For this review, take the finished solid that the model builds, in its own axes (mm). A direction names the side the tool comes from. Round coordinates to 2 decimals unless told otherwise and drop trailing zeros. Write each loop counter-clockwise with the first axis right and the second up, starting at its lowest first coordinate (ties: lowest second). Pieces come first, ordered by that corner, then holes. Notation, with made-up numbers: M 65.5,41.25 L 92.5,41.25 A22 ccw 92.5,70.25 Z; hole C 57,87 d10. An arc over 180 degrees is marked long. Answer in a Markdown table with one row per item.
```python
from build123d import *

# Parameters (mm, degrees)
SKETCH1_R           = 3.25
SKETCH1_R_2         = 2.25
BOSS_EXTRUDE1_DEPTH = 4.5
SKETCH2_R           = 8.5
SKETCH2_R_2         = 0.85
SKETCH2_R_3         = 1
BOSS_EXTRUDE2_DEPTH = 2


with BuildPart() as part:
    # Sketch1 → Boss-Extrude1 (new body)
    with BuildSketch(Plane.XY):
        Circle(SKETCH1_R)
        Circle(SKETCH1_R_2, mode=Mode.SUBTRACT)
    extrude(amount=BOSS_EXTRUDE1_DEPTH)

    # Sketch2 → Boss-Extrude2 (add)
    with BuildSketch(Plane(origin=(0, 0, 0), x_dir=(-1, 0, 0), z_dir=(0, 0, -1))):
        Circle(SKETCH2_R)
        Circle(SKETCH2_R_2, mode=Mode.SUBTRACT)
        with Locations((-6, 0)):
            Circle(SKETCH2_R_3, mode=Mode.SUBTRACT)
        with Locations((0, 6)):
            Circle(SKETCH2_R_3, mode=Mode.SUBTRACT)
        with Locations((6, 0)):
            Circle(SKETCH2_R_3, mode=Mode.SUBTRACT)
        with Locations((0, -6)):
            Circle(SKETCH2_R_3, mode=Mode.SUBTRACT)
    extrude(amount=-BOSS_EXTRUDE2_DEPTH)


solid = part.part
```
Q1. Take a section at A-A (y = -6). State the section outline as (x, z) points.
Found:
| item | result |
|---|---|
| outline | M -6.02,0 L -1,0 L -1,2 L -6.02,2 Z; M 1,0 L 6.02,0 L 6.02,2 L 1,2 Z |
Q2. Take a section at C-C (z = 0.75). State the section outline as (x, y) points, then the cut area to 3 significant figures.
Found:
| item | result |
|---|---|
| outline | C 0,0 d17; hole C -6,0 d2; hole C 0,-6 d2; hole C 0,6 d2; hole C 0,0 d1.7; hole C 6,0 d2 |
| area | 212 mm² |
Q3. Mouldability with a two-part tool opening along X and no side actions: class faces 3 (the face through (0, -5, 1)), 4 (the face through (-2.579, -1.978, 3.232)), 5 (the face through (-4, 0, 2)) as +X half, -X half, draft (parallel to the pull), parting line (faces both ways), or undercut.
Found:
| item | result |
|---|---|
| face 3 | undercut |
| face 4 | parting line |
| face 5 | draft |
Q4. Machinability: for faces 1 (the face through (6.8, -0.6, 1)), 2 (the face through (-0.29, 2.23, 3.23)), which of the approach directions +Z, -Z, +X, -X, +Y, -Y give a long, thin tool a straight path to every point of the face, cutting with its end or side? Answer none if there is none.
Found:
| item | result |
|---|---|
| face 1 | +Z, -Z |
| face 2 | +Z |
Q5. For probe 1 along Y at (x, z) = (0, 0.7); probe 2 along X at (y, z) = (0, 3.45), list the stretches that pass through material, from the lowest coordinate up.
Found:
| item | result |
|---|---|
| probe 1 | -8.5 to -7, -5 to -0.85, 0.85 to 5, 7 to 8.5 |
| probe 2 | -3.25 to -2.25, 2.25 to 3.25 |
Q6. Insertion check: P1, Ø3, axis at x = 0, y = 6, coming from the +Z side. The pin has a flat end and moves straight along its axis. Give the tip position at first contact, or say it passes through.
Found:
| item | result |
|---|---|
| P1 | z = 2 |
Q7. Take a section at D-D (y = -0.25). State the section outline as (x, z) points, then the cut area to 3 significant figures.
Found:
| item | result |
|---|---|
| outline | M -8.5,0 L -6.97,0 L -6.97,2 L -8.5,2 Z; M -5.03,0 L -0.81,0 L -0.81,2 L -2.24,2 L -2.24,4.5 L -3.24,4.5 L -3.24,2 L -5.03,2 Z; M 0.81,0 L 5.03,0 L 5.03,2 L 3.24,2 L 3.24,4.5 L 2.24,4.5 L 2.24,2 L 0.81,2 Z; M 6.97,0 L 8.5,0 L 8.5,2 L 6.97,2 Z |
| area | 28.0 mm² |
